For this review, use the dimensioned drawing (mm, ordinates from the lowest corner) and the shaded views. Round coordinates to 2 decimals unless told otherwise and drop trailing zeros. Write each loop counter-clockwise with the first axis right and the second up, starting at its lowest first coordinate (ties: lowest second). Pieces come first, ordered by that corner, then holes. Notation, with made-up numbers: (31.25, 75) - (38.25, 75) arc R20 cw to (38.25, 87) - close; hole circle Ø7 at (56.25, 77.25). An arc over 180 degrees is marked (long way). Return JSON: item names as keys, results as strings.
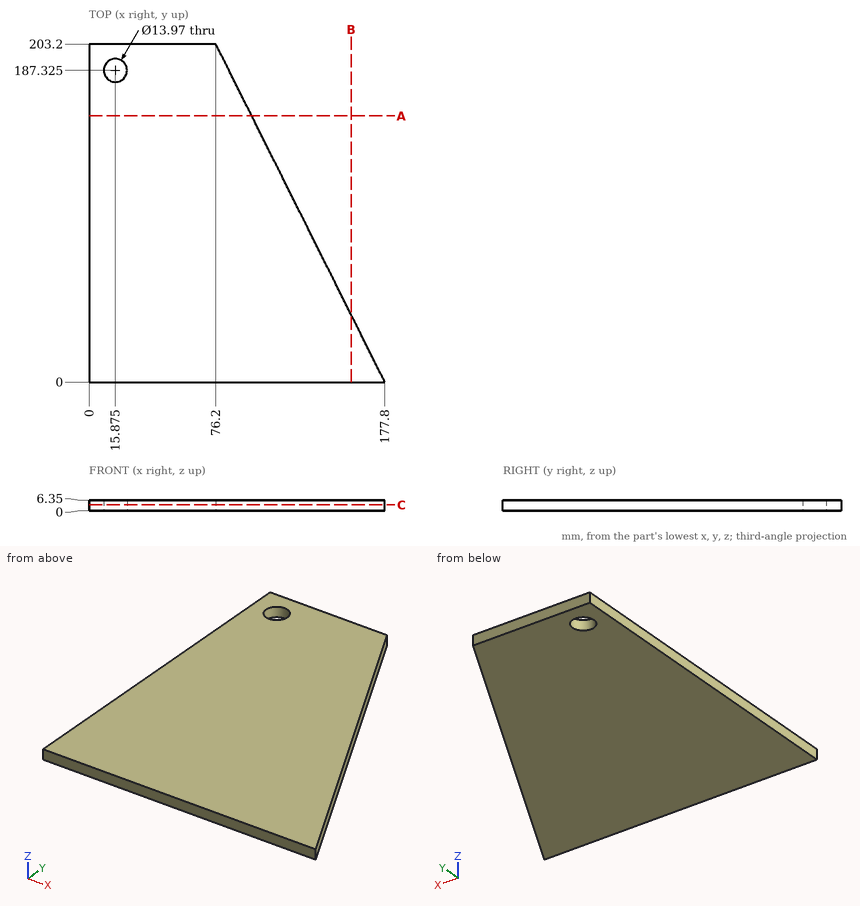
(1) Add section A-A (y = 160). Write out the cut boundary in (x, z), plus the area to 3 significant figures.
Filled in:
{"outline": "(0, 0) - (97.8, 0) - (97.8, 6.35) - (0, 6.35) - close", "area": "621 mm2"}
(2) Add section C-C (z = 3.5). Write out the cut boundary in (x, y) (3 decimals), plus the area to 3 significant figures.
Filled in:
{"outline": "(0, 0) - (177.8, 0) - (76.2, 203.2) - (0, 203.2) - close; hole circle Ø13.97 at (15.875, 187.325)", "area": "25,700 mm2"}
(3) Wall thickness on line 1 (X direction, y = 136, z = 4.25); line 2 (X direction, y = 80, z = 1.5); line 3 (Y direction, x = 85, z = 3.5): over which ranges is each line inside the solid? List them lowest first.
Filled in:
{"line 1": "x = 0 to 109.8", "line 2": "x = 0 to 137.8", "line 3": "y = 0 to 185.6"}
(4) Clearance check with a flat-ended pin moving along its axis: pin 1 Ø8.5 at (x, y) = (15.875, 187.325) entering from -Z. State where the tip first meets the part, or that it passes through.
Filled in:
{"pin 1": "passes through"}
(5) Add section B-B (x = 157.5). Write out the cut boundary in (y, z).
Filled in:
{"outline": "(0, 0) - (40.6, 0) - (40.6, 6.35) - (0, 6.35) - close"}
